Read the model definition and answer for the solid it produces. Units are mm, in the model's axes. Face numbers are marked on the shaded views. A direction names the side the tool comes from. Coordinates: 2 decimals unless noted, no trailing zeros. Write each loop counter-clockwise with the first axis right and the second up, starting at its lowest first coordinate (ties: lowest second). Pieces come first, ordered by that corner, then holes. Notation, with made-up numbers: M -6,-22.75 L 10,-22.75 A7 ccw 10,-9.75 Z; hole C -27,3.25 d8. An arc over 180 degrees is marked long. Write item = value, one per line.
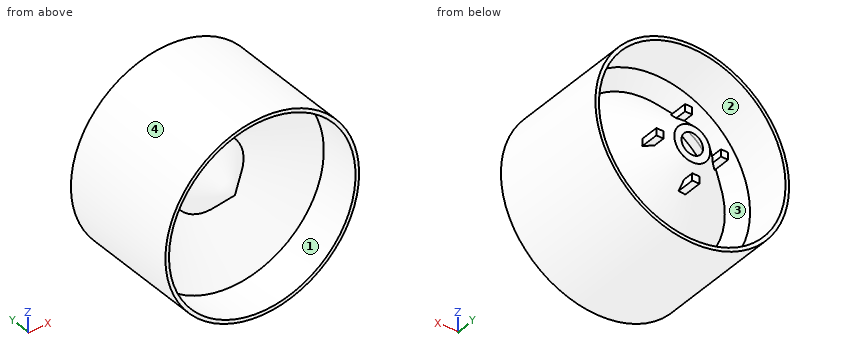
Autodesk Inventor part; units mm, degrees
ref_plane "YZ Plane" through (0, 0, 0) normal (1, 0, 0) x (0, 1, 0)
ref_plane "XZ Plane" through (0, 0, 0) normal (0, 1, 0) x (-1, 0, 0)
ref_plane "XY Plane" through (0, 0, 0) normal (0, 0, 1) x (1, 0, 0)
sketch "Sketch1" plane through (0, 0, 0) normal (0, 0, 1) x (1, 0, 0)
  line L0 (-3.313, 2.109) -> (-3.313, 22.109)
  line L1 (-3.313, 4.109) -> (-3.313, 2.109)
  line L2 (22.687, -0.5116) -> (12.687, 9.4884)
  line L3 (12.687, 9.4884) -> (12.687, 7.4884)
  line L4 (12.687, 7.4884) -> (22.687, -2.5116)
  line L5 (22.687, -2.5116) -> (22.687, -0.5116)
  line L6 (-0.313, 2.109) -> (19.687, 22.109)
  line L7 (19.687, 22.109) -> (17.687, 22.109)
  line L8 (17.687, 22.109) -> (-0.313, 4.109)
  line L9 (12.187, 14.609) -> (13.6012, 16.0232)
  line L10 (-0.313, 2.109) -> (19.687, 22.109)
  line L11 (17.687, 22.109) -> (-0.313, 4.109)
  line L12 (-0.313, 4.109) -> (-0.313, 2.109)
  line L13 (19.687, 22.109) -> (17.687, 22.109)
  line L14 (-0.313, 4.109) -> (-0.313, 2.109)
  line L15 (-0.313, 2.109) -> (19.687, 22.109)
  line L16 (17.687, 22.109) -> (-0.313, 4.109)
  line L17 (-0.313, 4.109) -> (-3.313, 7.109)
  line L18 (-3.313, 22.109) -> (-4.313, 22.109)
  line L19 (-3.313, 7.109) -> (-3.313, 9.109)
  line L20 (-3.313, 9.109) -> (0.687, 5.109)
  line L21 (-3.313, 7.109) -> (-3.313, -2.5116)
  line L22 (-4.313, -2.5116) -> (-4.313, 22.109)
  line L23 (-3.313, 22.109) -> (-3.313, 9.109)
  line L24 (-4.313, -2.5116) -> (-3.313, -2.5116)
  line L25 (-4.313, -2.5116) -> (-4.313, -12.5116)
  line L26 (-4.313, -12.5116) -> (-3.313, -12.5116)
  line L27 (-3.313, -12.5116) -> (-3.313, -2.5116)
  line L28 (-0.313, 2.109) -> (-3.313, -0.891)
  line L29 (-3.313, 1.109) -> (-0.313, 4.109)
  dimension "d20" = 2
  dimension "d21" = 2
  dimension "d50" = 1
  dimension "d67" = 23
  dimension "d69" = 2
  dimension "d71" = 10
revolve "Revolution4" add sketch "Sketch1" angle 360 about axis through (22.687, -2.5116, 0) along (0, 1, 0) contours L8 L7 L6 L12
sketch "Sketch2" plane through (22.687, 22.109, 0) normal (0, 1, 0) x (1, 0, 0)
  circle A0 centre (0, 0) radius 3
  circle A1 centre (0, 0) radius 10
  line L0 (0, 0) -> (10, 0)
  circle A2 centre (0, 0) radius 10
  line L1 (0, 0) -> (0, -10)
  line L2 (0, 0) -> (0, -10)
  line L3 (0, 0) -> (-10, 0)
  line L4 (0, 0) -> (0, 10)
  line L5 (0, -8) -> (0, -10)
  line L6 (0, -8) -> (0, -10)
  line L7 (10, 0) -> (8, 0)
  line L8 (8, 0) -> (8, 2)
  line L9 (8, 2) -> (10, 2)
  line L10 (10, 2) -> (10, 0)
  line L11 (0, 8) -> (0, 10)
  line L12 (-10, 0) -> (-8, 0)
  line L13 (-8, 0) -> (-8, -2)
  line L14 (-8, -2) -> (-10, -2)
  line L15 (-10, -2) -> (-10, 0)
  line L16 (0, 8) -> (0, 10)
  line L17 (0, 8) -> (-2, 8)
  line L18 (-2, 8) -> (-2, 10)
  line L19 (-2, 10) -> (0, 10)
  line L20 (0, 10) -> (0, 8)
  line L21 (0, -10) -> (2, -10)
  line L22 (2, -10) -> (2, -8)
  line L23 (2, -8) -> (0, -8)
  line L24 (0, -8) -> (0, -10)
  point P0 (-22.687, 0)
  dimension "d29" = 20
  dimension "d34" = 2
  dimension "d35" = 2
  dimension "d54" = 2
  dimension "d56" = 2
  dimension "d57" = 2
revolve "Revolution10" add sketch "Sketch1" angle 360 about axis through (22.687, -2.5116, 0) along (0, 1, 0) contours L5 L4 L3 L2
extrude "Extrusion5" add sketch "Sketch2" against normal blind 14 contours L17 L18 A1 L4 | A1 L18 L19
extrude "Extrusion6" add sketch "Sketch2" against normal blind 14 contours L23 L22 A1 L1 | A1 L22 L21
extrude "Extrusion7" add sketch "Sketch2" against normal blind 14 contours L13 L14 A1 L3 | A1 L14 L15
extrude "Extrusion8" add sketch "Sketch2" against normal blind 14 contours L8 L9 A1 L0 | A1 L9 L10
revolve "Revolution11" add sketch "Sketch1" angle 360 about axis through (22.687, -2.5116, 0) along (0, 1, 0) contours L21 L24 L22 L18 L0 | L0 L20 L8 L17
sketch "Sketch3" plane through (22.687, -2.5116, 0) normal (0, -1, 0) x (1, 0, 0)
  point P0 (-22.687, 0)
revolve "Revolution12" add sketch "Sketch1" angle 360 about axis through (22.687, -2.5116, 0) along (0, 1, 0) contours L21 L24 L22 L18 L0 | L29 L12 L28 L21 | L27 L26 L25 L24
properties part number "flyflipfunnel"
Item 1: For a pull along Z with two mould halves and no side action, classify the marked faces 3 and 4 as released by +Z, released by -Z, zero draft, split by the parting line, or undercut.
Worked answers:
face_3 = undercut
face_4 = split by the parting line
Item 2: Which of the six approach directions +Z, -Z, +X, -X, +Y, -Y give full straight-line access (tool end or side, diameter ignored) to the marked faces 1 and 2?
Worked answers:
face_1 = -Y
face_2 = +Y
Item 3: Find section A-A (y = 18). Determine the outline of the cut face in (x, z).
Worked answers:
outline = C 22.69,0 d54; M 12.69,0 L 13.58,0 A9.11 ccw 20.69,-8.89 L 20.69,-10 L 22.69,-10 L 22.69,-9.11 A9.11 ccw 31.57,-2 L 32.69,-2 L 32.69,0 L 31.8,0 A9.11 ccw 24.69,8.89 L 24.69,10 L 22.69,10 L 22.69,9.11 A9.11 ccw 13.8,2 L 12.69,2 Z; hole C 22.69,0 d52; hole C 22.69,0 d14.22
Item 4: Flat-ended cylindrical pins translate along their axes: pin 1 (5 mm diameter, centred on y = 11.5, z = -21, fed in from -X); pin 2 (1 mm diameter, centred on x = 9, z = -18, fed in from +Y); pin 3 (2 mm diameter, centred on y = 14, z = -9.5, fed in from +X). Find the tip coordinate at first contact, or state that the pin passes through.
Worked answers:
pin_1 = 3.02
pin_2 = 6.22
pin_3 = 48.31
Item 5: Consider line 1 along Z through (x, y) = (29, 12.5); line 2 along Z through (x, y) = (19, 13); line 3 along Z through (x, y) = (23, -9). Determine where each line is inside the solid, lowest interval first. Write a range as from..to.
Worked answers:
line_1 = -26.25..-25.22, -13.17..-10.91, 10.91..13.17, 25.22..26.25
line_2 = -26.75..-25.74, -13.62..-11.53, 11.53..13.62, 25.74..26.75
line_3 = -27..-26, 26..27
Item 6: Find section B-B (y = -4). Determine the outline of the cut face in (x, z).
Worked answers:
outline = C 22.69,0 d54; hole C 22.69,0 d52
Item 7: Find section C-C (z = 15.5). State how many separate pieces and enclosed holes the cut face has, and give its area (3 significant figures).
Worked answers:
separate_pieces = 1
enclosed_holes = 2
area = 187 mm²
